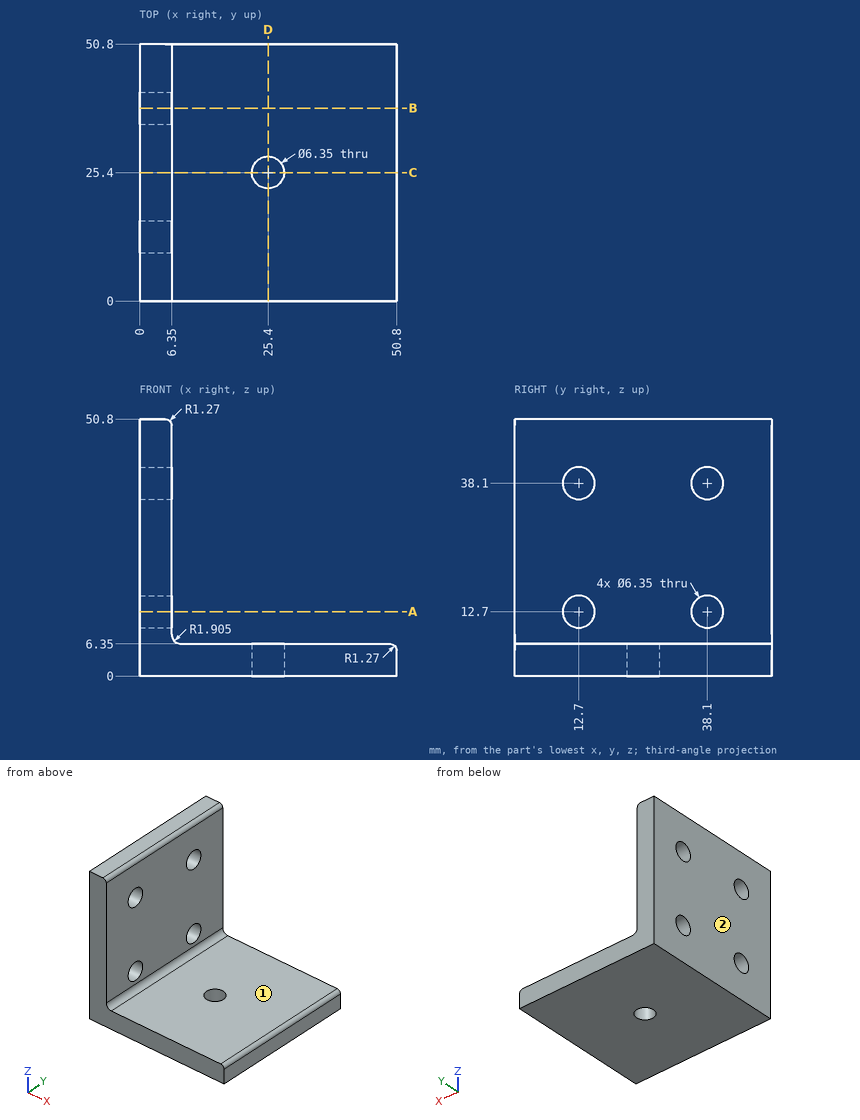
Input: dimensioned drawing with shaded views. Units: mm. Origin: part minimum x, y, z. A direction names the side the tool comes from. Give positions to 0.01 mm unless a question says otherwise; leave off trailing zeros. Order: outer loops, then holes, each group sorted by start corner. A loop starts at its lowest first (then second) coordinate and runs counter-clockwise, first axis right, second up. Notation, with made-up numbers: (-23, 75.25) -> (-16, 75.25) arc R8 cw to (-16, 82.25) -> close; hole circle Ø2 at (56, -23). An arc over 180 degrees is marked (long way). Use one line per item in the form item = value.
1) Section D-D, the plane x = 25.4. Return loops of the section in (y, z) (3 decimals).
Response values:
outline = (0, 0) -> (22.225, 0) -> (22.225, 6.35) -> (0, 6.35) -> close; (28.575, 0) -> (50.8, 0) -> (50.8, 6.35) -> (28.575, 6.35) -> close
2) Reachability of the marked faces 1 and 2 from +Z, -Z, +X, -X, +Y, -Y: full face, straight path, thin tool, end or side. Return the list, or none.
Response values:
face_1 = +Z, +X, +Y, -Y
face_2 = +Z, -Z, -X, +Y, -Y
3) First-contact query: pin 1 Ø12.5 at (x, y) = (37.5, 13.5) entering from +Z; pin 2 Ø2 at (y, z) = (42, 16) entering from +X. Flat tips, straight axial feed; report the tip coordinate or a pass-through.
Response values:
pin_1 = 6.35
pin_2 = 6.35
4) Line query: probe 1 along Z at (x, y) = (4, 38); probe 2 along Y at (x, z) = (25.4, 2) (3 decimals). Output: solid intervals per line, ascending.
Response values:
probe_1 = 0 to 9.53, 15.87 to 34.93, 41.27 to 50.8
probe_2 = 0 to 22.225, 28.575 to 50.8
5) Section C-C, the plane y = 25.4. Return loops of the section in (x, z) (3 decimals), and give its area (3 significant figures).
Response values:
outline = (0, 0) -> (22.225, 0) -> (22.225, 6.35) -> (8.255, 6.35) arc R1.905 cw to (6.35, 8.255) -> (6.35, 49.53) arc R1.27 ccw to (5.08, 50.8) -> (0, 50.8) -> close; (28.575, 0) -> (50.8, 0) -> (50.8, 5.08) arc R1.27 ccw to (49.53, 6.35) -> (28.575, 6.35) -> close
area = 565 mm^2
6) Section B-B, the plane y = 38.1. Return loops of the section in (x, z) (3 decimals).
Response values:
outline = (0, 0) -> (50.8, 0) -> (50.8, 5.08) arc R1.27 ccw to (49.53, 6.35) -> (8.255, 6.35) arc R1.905 cw to (6.35, 8.255) -> (6.35, 9.525) -> (0, 9.525) -> close; (0, 15.875) -> (6.35, 15.875) -> (6.35, 34.925) -> (0, 34.925) -> close; (0, 41.275) -> (6.35, 41.275) -> (6.35, 49.53) arc R1.27 ccw to (5.08, 50.8) -> (0, 50.8) -> close
7) Section A-A, the plane z = 12.7. Return loops of the section in (x, y) (3 decimals).
Response values:
outline = (0, 0) -> (6.35, 0) -> (6.35, 9.525) -> (0, 9.525) -> close; (0, 15.875) -> (6.35, 15.875) -> (6.35, 34.925) -> (0, 34.925) -> close; (0, 41.275) -> (6.35, 41.275) -> (6.35, 50.8) -> (0, 50.8) -> close
